Can you work these out from the model? Positions are in its coordinate system, mm. A direction names the side the tool comes from. Give positions to 0.01 mm unless a question says otherwise; leave off trailing zeros. Write each loop counter-clockwise with the first axis right and the second up, starting at its lowest first coordinate (ties: lowest second). Pieces come first, ordered by that corner, then holes. Notation, with made-up numbers: M 18,58 L 47,58 A21 ccw 47,64 Z; hole C 47,-17 d11. An arc over 180 degrees is marked long. Write each question's results on one line, items separated by ' | '.
Solid Edge part; units mm, degrees
sketch "Sketch1" plane through (0, 0, 0) normal (0, 0, 1) x (1, 0, 0)
  line L0 (-125, -180) -> (125, -180)
  line L1 (125, -180) -> (125, 180)
  line L2 (125, 180) -> (-125, 180)
  line L3 (-125, 180) -> (-125, -180)
extrude "Protrusion1" add sketch "Sketch1" along normal blind 7
sketch "Sketch2" plane through (0, 0, 7) normal (0, 0, 1) x (1, 0, 0)
  line L0 (75, -180) -> (-75, -180)
  arc A0 (-125, -130) -> (-75, -180) centre (-75, -130) ccw
  line L1 (-125, -130) -> (-125, 130)
  arc A1 (-125, 130) -> (-75, 180) centre (-75, 130) cw
  line L2 (-75, 180) -> (75, 180)
  arc A2 (125, 130) -> (75, 180) centre (75, 130) ccw
  line L3 (125, 130) -> (125, -130)
  arc A3 (125, -130) -> (75, -180) centre (75, -130) cw
  line L4 (75, 170) -> (-75, 170)
  arc A4 (-115, 130) -> (-75, 170) centre (-75, 130) cw
  line L5 (-115, 130) -> (-115, -130)
  arc A5 (-115, -130) -> (-75, -170) centre (-75, -130) ccw
  line L6 (-75, -170) -> (75, -170)
  arc A6 (115, -130) -> (75, -170) centre (75, -130) cw
  line L7 (115, -130) -> (115, 130)
  arc A7 (115, 130) -> (75, 170) centre (75, 130) ccw
extrude "ExtrudedProtrusion_3" add sketch "Sketch2" along normal blind 10
sketch "Sketch3" plane through (0, 0, 17) normal (0, 0, 1) x (1, 0, 0)
  line L0 (-42.5, -180) -> (42.5, -180)
  line L1 (42.5, -180) -> (42.5, 180)
  line L2 (42.5, 180) -> (-42.5, 180)
  line L3 (-42.5, 180) -> (-42.5, -180)
extrude "ExtrudedCutout_1" cut sketch "Sketch3" against normal blind 10
sketch "Sketch4" plane through (0, 0, 0) normal (0, 0, -1) x (1, 0, 0)
  line L0 (125, -180) -> (-125, -180)
  line L1 (-125, -180) -> (-125, 180)
  line L2 (-125, 180) -> (125, 180)
  line L3 (125, 180) -> (125, -180)
extrude "ExtrudedProtrusion_4" add sketch "Sketch4" along normal blind 25
Item 1: I want a section at C-C, the plane y = -138. Please give me the cut outline in (x, z), and give its area (3 significant figures).
Geometry says:
outline: M -125,-25 L 125,-25 L 125,7 L 124.36,7 L 124.36,17 L 114.19,17 L 114.19,7 L -114.19,7 L -114.19,17 L -124.36,17 L -124.36,7 L -125,7 Z | area: 8,200 mm2
Item 2: I want a section at B-B, the plane x = 105.5. Please give me the cut outline in (y, z), and give its area (3 significant figures).
Geometry says:
outline: M -180,-25 L 180,-25 L 180,7 L 169.62,7 L 169.62,17 L 155.88,17 L 155.88,7 L -155.88,7 L -155.88,17 L -169.62,17 L -169.62,7 L -180,7 Z | area: 11,800 mm2
Item 3: I want a section at A-A, the plane y = 63.5. Please give me the cut outline in (x, z).
Geometry says:
outline: M -125,-25 L 125,-25 L 125,17 L 115,17 L 115,7 L -115,7 L -115,17 L -125,17 Z
Item 4: If I drill on line 1 (Z direction, x = -93, y = -139.5); line 2 (Y direction, x = 44.5, z = 15); line 3 (Y direction, x = -100.5, z = 10), over which ranges is the centre line in solid material (lowest first)? Write a range as from..to.
Geometry says:
line 1: z = -25..7 | line 2: y = -180..-170, 170..180 | line 3: y = -173.01..-160.82, 160.82..173.01
Item 5: For faces 1 (the face through (-109.964, -165.742, 11.93)), 2 (the face through (2, 180, -9)), 3 (the face through (-115, 168, 7)), 4 (the face through (115, -170, 7)), 5 (the face through (-59, 170, 12)), which set-ups out of +Z, -Z, +X, -X, +Y, -Y let a thin tool reach every point of the face, with its end or its side?
Geometry says:
face 1: +Z, -X, -Y | face 2: +Z, -Z, +X, -X, +Y | face 3: +Z, -X, +Y | face 4: +Z, +X, -Y | face 5: +Z
Item 6: I'm going to push flat-ended pins straight in: pin 1 (2 mm diameter, centred on x = 21.5, y = 63.5, fed in from +Z); pin 2 (3 mm diameter, centred on y = -176, z = 10, fed in from -X); pin 3 (5 mm diameter, centred on y = -174.5, z = 10.5, fed in from +X). Where does each tip first touch, or does it pass through?
Geometry says:
pin 1: stops at z = 7 | pin 2: stops at x = -97.8 | pin 3: stops at x = 102.13
Item 7: Thinking about a two-plate mould opening in X: for faces 6 (the face through (-115, -168, 7)), 7 (the face through (115, -2, 12)), 8 (the face through (-59, -170, 12)), 9 (the face through (109.964, 165.742, 11.93)), which applies, +X half, -X half, draft (parallel to the pull), parting line (faces both ways), or undercut?
Geometry says:
face 6: draft | face 7: undercut | face 8: undercut | face 9: +X half
Item 8: I want a section at D-D, the plane x = -38.5. Please give me the cut outline in (y, z).
Geometry says:
outline: M -180,-25 L 180,-25 L 180,7 L -180,7 Z
